Source: CAD feature listing. Evaluate the final solid. Frame: model axes, mm. A direction names the side the tool comes from. Round coordinates to 2 decimals unless told otherwise and drop trailing zeros. Loops run counter-clockwise (first coordinate to the right, second up) from the corner with the lowest first, then second, coordinate; pieces in that order, holes last. Notation, with made-up numbers: M -11,77 L 29,77 A37 ccw 29,115 Z; hole C -23.75,10 d9. An arc over 180 degrees is marked long. One line per item, written item: value.
from build123d import *

# Parameters (mm, degrees)
F0_R         = 15
F1_DEPTH     = 100
F2_T1_DEPTH  = 180
F2_T3_DEPTH  = 277.5790250274
F2_T5_DEPTH  = 80
F2_T7_DEPTH  = 279.8718117474
F2_T9_DEPTH  = 180.014601827
F2_S13_W     = 10
F2_S13_H     = 10
F2_T14_DEPTH = 10
F2_S19_W     = 10
F2_S19_H     = 10
F2_T20_DEPTH = 10
F2_T26_DEPTH = 10
F2_S31_W     = 10
F2_S31_H     = 10
F2_T32_DEPTH = 10
F2_T38_DEPTH = 10
F2_S43_W     = 10
F2_S43_H     = 10
F2_T44_DEPTH = 10
F2_T50_DEPTH = 10
F2_T56_DEPTH = 10


# Not quite as in the source:
# - a fillet or chamfer that OpenCascade refuses, or shapes differently, is made with other operations: its cross-section is extruded or revolved along the edge and cut away or added


with BuildPart() as f1:
    # F0 (on Top) → F1 (new body)
    with BuildSketch(Plane.XY):
        Polygon((148.6140583592, 151.6970589757), (-151.3859416408, 151.6970589757), (-148.8384008408, -48.3029410243), (148.6140583592, -48.3029410243), align=None)
        with Locations((124.343521893, 52.9859960079)):
            Circle(F0_R, mode=Mode.SUBTRACT)
    extrude(amount=F1_DEPTH)

    # F2: fillet of radius 10 on 12 edges, made by hand

    # F2_s2 → F2_t1 (cut)
    with BuildSketch(Plane.XZ.offset(-141.6970589757)):
        with BuildLine():
            ThreePointArc((148.6140583592, 90), (145.6851261711, 97.0710678119), (138.6140583592, 100))
            Line((138.6140583592, 100), (148.6140583592, 100))
            Line((148.6140583592, 100), (148.6140583592, 90))
        make_face()
        with BuildLine():
            ThreePointArc((148.6140583592, 10), (145.6851261711, 2.9289321881), (138.6140583592, 0))
            Line((138.6140583592, 0), (148.6140583592, 0))
            Line((148.6140583592, 0), (148.6140583592, 10))
        make_face()
    extrude(amount=F2_T1_DEPTH, mode=Mode.SUBTRACT)

    # F2_s4 → F2_t3 (cut)
    with BuildSketch(Plane.YZ.offset(-138.9649666681)):
        with BuildLine():
            ThreePointArc((-48.3029410243, 90), (-45.3740088362, 97.0710678119), (-38.3029410243, 100))
            Line((-38.3029410243, 100), (-48.3029410243, 100))
            Line((-48.3029410243, 100), (-48.3029410243, 90))
        make_face()
        with BuildLine():
            ThreePointArc((-48.3029410243, 10), (-45.3740088362, 2.9289321881), (-38.3029410243, 0))
            Line((-38.3029410243, 0), (-48.3029410243, 0))
            Line((-48.3029410243, 0), (-48.3029410243, 10))
        make_face()
    extrude(amount=F2_T3_DEPTH, mode=Mode.SUBTRACT)

    # F2_s6 → F2_t5 (cut)
    with BuildSketch(Plane.XY.offset(10)):
        with BuildLine():
            ThreePointArc((138.6140583592, -48.3029410243), (145.6851261711, -45.3740088362), (148.6140583592, -38.3029410243))
            Line((148.6140583592, -38.3029410243), (148.6140583592, -48.3029410243))
            Line((148.6140583592, -48.3029410243), (138.6140583592, -48.3029410243))
        make_face()
        with BuildLine():
            ThreePointArc((148.6140583592, 141.6970589757), (145.6851261711, 148.7681267876), (138.6140583592, 151.6970589757))
            Line((138.6140583592, 151.6970589757), (148.6140583592, 151.6970589757))
            Line((148.6140583592, 151.6970589757), (148.6140583592, 141.6970589757))
        make_face()
        with BuildLine():
            ThreePointArc((-138.9649666681, -48.3029410243), (-145.9908592421, -45.4188972875), (-148.9641555213, -38.4303077322))
            Line((-148.9641555213, -38.4303077322), (-148.8384008408, -48.3029410243))
            Line((-148.8384008408, -48.3029410243), (-138.9649666681, -48.3029410243))
        make_face()
        with BuildLine():
            ThreePointArc((-141.2577533882, 151.6970589757), (-148.3737096513, 148.7229515496), (-151.2569422414, 141.5696922678))
            Line((-151.2569422414, 141.5696922678), (-151.3859416408, 151.6970589757))
            Line((-151.3859416408, 151.6970589757), (-141.2577533882, 151.6970589757))
        make_face()
    extrude(amount=F2_T5_DEPTH, mode=Mode.SUBTRACT)

    # F2_s8 → F2_t7 (cut)
    with BuildSketch(Plane.YZ.offset(-141.2577533882)):
        with BuildLine():
            ThreePointArc((151.6970589757, 10), (148.7681267876, 2.9289321881), (141.6970589757, 0))
            Line((141.6970589757, 0), (151.6970589757, 0))
            Line((151.6970589757, 0), (151.6970589757, 10))
        make_face()
        with BuildLine():
            ThreePointArc((151.6970589757, 90), (148.7681267876, 97.0710678119), (141.6970589757, 100))
            Line((141.6970589757, 100), (151.6970589757, 100))
            Line((151.6970589757, 100), (151.6970589757, 90))
        make_face()
    extrude(amount=F2_T7_DEPTH, mode=Mode.SUBTRACT)

    # F2_s10 → F2_t9 (cut)
    with BuildSketch(Plane(origin=(-1.8275176256, 143.4730800475, 0), x_dir=(0, 0, 1), z_dir=(0.0127366708, -0.9999188853, 0))):
        with BuildLine():
            ThreePointArc((10, 149.4415465191), (2.9289321881, 146.512614331), (0, 139.4415465191))
            Line((0, 139.4415465191), (0, 149.4415465191))
            Line((0, 149.4415465191), (10, 149.4415465191))
        make_face()
        with BuildLine():
            ThreePointArc((90, 149.4415465191), (97.0710678119, 146.512614331), (100, 139.4415465191))
            Line((100, 139.4415465191), (100, 149.4415465191))
            Line((100, 149.4415465191), (90, 149.4415465191))
        make_face()
    extrude(amount=F2_T9_DEPTH, mode=Mode.SUBTRACT)


with BuildPart() as f2_tool12:
    # F2_s13 → F2_t14 (new body)
    with BuildSketch(Plane.XZ.offset(38.3029410243)):
        with Locations((143.6140583592, 95)):
            Rectangle(F2_S13_W, F2_S13_H)
    extrude(amount=F2_T14_DEPTH)

    # F2_s15 → F2_t16 (revolve, cut)
    with BuildSketch(Plane(origin=(138.6140583592, -38.3029410243, 90), x_dir=(-0.7071067812, 0, -0.7071067812), z_dir=(-0.7071067812, 0, 0.7071067812))):
        with BuildLine():
            ThreePointArc((0, -10), (10, 0), (0, 10))
            Line((0, 10), (0, -10))
        make_face()
    revolve(axis=Axis((138.6140583592, -38.3029410243, 90), (0, -1, 0)), mode=Mode.SUBTRACT)


with BuildPart() as f1_1:
    add(f1.part)

    # F2_t11: cut F2_tool12
    add(f2_tool12.part, mode=Mode.SUBTRACT)


with BuildPart() as f2_tool18:
    # F2_s19 → F2_t20 (new body)
    with BuildSketch(Plane.YZ.offset(138.6140583592)):
        with Locations((146.6970589757, 95)):
            Rectangle(F2_S19_W, F2_S19_H)
    extrude(amount=F2_T20_DEPTH)

    # F2_s21 → F2_t22 (revolve, cut)
    with BuildSketch(Plane(origin=(138.6140583592, 141.6970589757, 90), x_dir=(0, -0.7071067812, -0.7071067812), z_dir=(0, -0.7071067812, 0.7071067812))):
        with BuildLine():
            ThreePointArc((0, -10), (10, 0), (0, 10))
            Line((0, 10), (0, -10))
        make_face()
    revolve(axis=Axis((138.6140583592, 141.6970589757, 90), (1, 0, 0)), mode=Mode.SUBTRACT)


with BuildPart() as f1_2:
    add(f1_1.part)

    # F2_t17: cut F2_tool18
    add(f2_tool18.part, mode=Mode.SUBTRACT)


with BuildPart() as f2_tool24:
    # F2_s25 → F2_t26 (new body)
    with BuildSketch(Plane.XY.offset(90)):
        Polygon((-138.9649666681, -38.3029410243), (-138.9649666681, -48.3029410243), (-148.8384008408, -48.3029410243), (-148.9641555213, -38.4303077322), align=None)
    extrude(amount=F2_T26_DEPTH)

    # F2_s27 → F2_t28 (revolve, cut)
    with BuildSketch(Plane(origin=(-138.9649666681, -38.3029410243, 90), x_dir=(0.7025892574, 0.7115956263, 0), z_dir=(0.7115956263, -0.7025892574, 0))):
        with BuildLine():
            ThreePointArc((0, -10), (10, 0), (0, 10))
            Line((0, 10), (0, -10))
        make_face()
    revolve(axis=Axis((-138.9649666681, -38.3029410243, 90), (0, 0, 1)), mode=Mode.SUBTRACT)


with BuildPart() as f1_3:
    add(f1_2.part)

    # F2_t23: cut F2_tool24
    add(f2_tool24.part, mode=Mode.SUBTRACT)


with BuildPart() as f2_tool30:
    # F2_s31 → F2_t32 (new body)
    with BuildSketch(Plane.XZ.offset(38.3029410243)):
        with Locations((143.6140583592, 5)):
            Rectangle(F2_S31_W, F2_S31_H)
    extrude(amount=F2_T32_DEPTH)

    # F2_s33 → F2_t34 (revolve, cut)
    with BuildSketch(Plane(origin=(138.6140583592, -38.3029410243, 10), x_dir=(-0.7071067812, 0, 0.7071067812), z_dir=(0.7071067812, 0, 0.7071067812))):
        with BuildLine():
            ThreePointArc((0, -10), (10, 0), (0, 10))
            Line((0, 10), (0, -10))
        make_face()
    revolve(axis=Axis((138.6140583592, -38.3029410243, 10), (0, -1, 0)), mode=Mode.SUBTRACT)


with BuildPart() as f1_4:
    add(f1_3.part)

    # F2_t29: cut F2_tool30
    add(f2_tool30.part, mode=Mode.SUBTRACT)


with BuildPart() as f2_tool36:
    # F2_s37 → F2_t38 (new body)
    with BuildSketch(Plane.XY.offset(10)):
        Polygon((-138.9649666681, -38.3029410243), (-138.9649666681, -48.3029410243), (-148.8384008408, -48.3029410243), (-148.9641555213, -38.4303077322), align=None)
    extrude(amount=-F2_T38_DEPTH)

    # F2_s39 → F2_t40 (revolve, cut)
    with BuildSketch(Plane(origin=(-138.9649666681, -38.3029410243, 10), x_dir=(0.7025892574, 0.7115956263, 0), z_dir=(-0.7115956263, 0.7025892574, 0))):
        with BuildLine():
            ThreePointArc((0, -10), (10, 0), (0, 10))
            Line((0, 10), (0, -10))
        make_face()
    revolve(axis=Axis((-138.9649666681, -38.3029410243, 10), (0, 0, -1)), mode=Mode.SUBTRACT)


with BuildPart() as f1_5:
    add(f1_4.part)

    # F2_t35: cut F2_tool36
    add(f2_tool36.part, mode=Mode.SUBTRACT)


with BuildPart() as f2_tool42:
    # F2_s43 → F2_t44 (new body)
    with BuildSketch(Plane.YZ.offset(138.6140583592)):
        with Locations((146.6970589757, 5)):
            Rectangle(F2_S43_W, F2_S43_H)
    extrude(amount=F2_T44_DEPTH)

    # F2_s45 → F2_t46 (revolve, cut)
    with BuildSketch(Plane(origin=(138.6140583592, 141.6970589757, 10), x_dir=(0, -0.7071067812, 0.7071067812), z_dir=(0, 0.7071067812, 0.7071067812))):
        with BuildLine():
            ThreePointArc((0, -10), (10, 0), (0, 10))
            Line((0, 10), (0, -10))
        make_face()
    revolve(axis=Axis((138.6140583592, 141.6970589757, 10), (1, 0, 0)), mode=Mode.SUBTRACT)


with BuildPart() as f1_6:
    add(f1_5.part)

    # F2_t41: cut F2_tool42
    add(f2_tool42.part, mode=Mode.SUBTRACT)


with BuildPart() as f2_tool48:
    # F2_s49 → F2_t50 (new body)
    with BuildSketch(Plane.XY.offset(10)):
        Polygon((-141.2577533882, 141.6970589757), (-141.2577533882, 151.6970589757), (-151.3859416408, 151.6970589757), (-151.2569422414, 141.5696922678), align=None)
    extrude(amount=-F2_T50_DEPTH)

    # F2_s51 → F2_t52 (revolve, cut)
    with BuildSketch(Plane(origin=(-141.2577533882, 141.6970589757, 10), x_dir=(0.7115956263, -0.7025892574, 0), z_dir=(0.7025892574, 0.7115956263, 0))):
        with BuildLine():
            ThreePointArc((0, -10), (10, 0), (0, 10))
            Line((0, 10), (0, -10))
        make_face()
    revolve(axis=Axis((-141.2577533882, 141.6970589757, 10), (0, 0, -1)), mode=Mode.SUBTRACT)


with BuildPart() as f1_7:
    add(f1_6.part)

    # F2_t47: cut F2_tool48
    add(f2_tool48.part, mode=Mode.SUBTRACT)


with BuildPart() as f2_tool54:
    # F2_s55 → F2_t56 (new body)
    with BuildSketch(Plane.XY.offset(90)):
        Polygon((-141.2577533882, 141.6970589757), (-141.2577533882, 151.6970589757), (-151.3859416408, 151.6970589757), (-151.2569422414, 141.5696922678), align=None)
    extrude(amount=F2_T56_DEPTH)

    # F2_s57 → F2_t58 (revolve, cut)
    with BuildSketch(Plane(origin=(-141.2577533882, 141.6970589757, 90), x_dir=(0.7115956263, -0.7025892574, 0), z_dir=(-0.7025892574, -0.7115956263, 0))):
        with BuildLine():
            ThreePointArc((0, -10), (10, 0), (0, 10))
            Line((0, 10), (0, -10))
        make_face()
    revolve(axis=Axis((-141.2577533882, 141.6970589757, 90), (0, 0, 1)), mode=Mode.SUBTRACT)


with BuildPart() as f1_8:
    add(f1_7.part)

    # F2_t53: cut F2_tool54
    add(f2_tool54.part, mode=Mode.SUBTRACT)


solid = f1_8.part
1. Ray query, line 1 (X direction, y = 139, z = 28); line 2 (X direction, y = 53.5, z = 73.5); line 3 (X direction, y = 50, z = 34). Return the intervals inside material, ascending. Write a range as [from, to].
Report:
line 1: x = [-151.22, 148.61]
line 2: x = [-150.14, 109.35], [139.33, 148.61]
line 3: x = [-150.09, 109.64], [139.04, 148.61]
2. Section query A-A (z = 29). Return the cut outline in (x, y), and give its area (3 significant figures).
Report:
outline: M -151.26,141.57 L -148.96,-38.43 A10 ccw -138.96,-48.3 L 138.61,-48.3 A10 ccw 148.61,-38.3 L 148.61,141.7 A10 ccw 138.61,151.7 L -141.26,151.7 A10 ccw Z; hole C 124.34,52.99 d30
area: 59,000 mm2
3. Reachability of faces 1 (the face through (145.76, 148.69, 49.44)), 2 (the face through (-147.28, 52.87, 96.99)) from +Z, -Z, +X, -X, +Y, -Y: full face, straight path, thin tool, end or side. Return the list, or none.
Report:
face 1: +Z, -Z, +X, +Y
face 2: +Z, -X, -Y
4. Pin query (flat end, axial travel): pin 1 (2 mm diameter, centred on y = 82, z = 59, fed in from -X). Return the tip coordinate at first contact, or that it passes through.
Report:
pin 1: stops at x = -150.51
5. Section query B-B (z = 93.5). Return the cut outline in (x, y) (1 decimal).
Report:
outline: M -150.6,141.6 L -148.3,-38.4 A9.4 ccw -139,-47.7 L 138.6,-47.7 A9.4 ccw 148,-38.3 L 148,141.7 A9.4 ccw 138.6,151.1 L -141.3,151.1 A9.4 ccw Z; hole C 124.3,53 d30
6. Pull-direction query (X, two-part tool) for faces 3 (the face through (-3.28, 148.85, 3.01)), 4 (the face through (-147.28, 52.87, 3.01)), 5 (the face through (138.2, 47.24, 49.3)); classes: released by +X, released by -X, zero draft, split by the parting line, or undercut.
Report:
face 3: zero draft
face 4: released by -X
face 5: undercut
